```python
from build123d import *

# Parameters (mm, degrees)
F0_W     = 115
F0_H     = 47
F1_DEPTH = 183
F2_W     = 95
F2_H     = 27
F2_R     = 8
F3_DEPTH = 2
F4_W     = 20
F4_H     = 3
F5_DEPTH = 183.001
F6_W     = 3
F6_H     = 13
F7_DEPTH = 47.001


with BuildPart() as f1:
    # F0 (on Top) → F1 (new body)
    with BuildSketch(Plane.XY):
        Rectangle(F0_W, F0_H)
    extrude(amount=F1_DEPTH)

    # F2 (on face) → F3 (cut)
    with BuildSketch(Plane.XY.offset(183)):
        Rectangle(F2_W, F2_H)
        with Locations((-31, 0)):
            Circle(F2_R, mode=Mode.SUBTRACT)
        with Locations((31, 0)):
            Circle(F2_R, mode=Mode.SUBTRACT)
    extrude(amount=-F3_DEPTH, mode=Mode.SUBTRACT)

    # F4 (on face) → F5 (cut, through all)
    with BuildSketch(Plane.XY.offset(183)):
        with Locations((-37.5, 22)):
            Rectangle(F4_W, F4_H)
        with Locations((-12.5, 22)):
            Rectangle(F4_W, F4_H)
        with Locations((12.5, 22)):
            Rectangle(F4_W, F4_H)
        with Locations((37.5, 22)):
            Rectangle(F4_W, F4_H)
        with Locations((37.5, -22)):
            Rectangle(F4_W, F4_H)
        with Locations((12.5, -22)):
            Rectangle(F4_W, F4_H)
        with Locations((-12.5, -22)):
            Rectangle(F4_W, F4_H)
        with Locations((-37.5, -22)):
            Rectangle(F4_W, F4_H)
    extrude(amount=-F5_DEPTH, mode=Mode.SUBTRACT)

    # F6 (on face) → F7 (cut, through all)
    with BuildSketch(Plane.XZ.offset(23.5)):
        with Locations((-56, 171.5)):
            Rectangle(F6_W, F6_H)
        with Locations((-56, 151.5)):
            Rectangle(F6_W, F6_H)
        with Locations((-56, 131.5)):
            Rectangle(F6_W, F6_H)
        with Locations((-56, 111.5)):
            Rectangle(F6_W, F6_H)
        with Locations((-56, 91.5)):
            Rectangle(F6_W, F6_H)
        with Locations((-56, 71.5)):
            Rectangle(F6_W, F6_H)
        with Locations((-56, 51.5)):
            Rectangle(F6_W, F6_H)
        with Locations((-56, 31.5)):
            Rectangle(F6_W, F6_H)
        with Locations((-56, 11.5)):
            Rectangle(F6_W, F6_H)
        with Locations((56, 171.5)):
            Rectangle(F6_W, F6_H)
        with Locations((56, 151.5)):
            Rectangle(F6_W, F6_H)
        with Locations((56, 131.5)):
            Rectangle(F6_W, F6_H)
        with Locations((56, 111.5)):
            Rectangle(F6_W, F6_H)
        with Locations((56, 91.5)):
            Rectangle(F6_W, F6_H)
        with Locations((56, 11.5)):
            Rectangle(F6_W, F6_H)
        with Locations((56, 51.5)):
            Rectangle(F6_W, F6_H)
        with Locations((56, 71.5)):
            Rectangle(F6_W, F6_H)
        with Locations((56, 31.5)):
            Rectangle(F6_W, F6_H)
    extrude(amount=-F7_DEPTH, mode=Mode.SUBTRACT)


solid = f1.part
```
Part model, mm, in its own coordinate system. A direction names the side the tool comes from. Give positions to 0.01 mm unless a question says otherwise; leave off trailing zeros. Write each loop counter-clockwise with the first axis right and the second up, starting at its lowest first coordinate (ties: lowest second). Pieces come first, ordered by that corner, then holes. Notation, with made-up numbers: (-36.75, 71.25) -> (9.25, 71.25) arc R25 ccw to (9.25, 93.25) -> close; hole circle Ø6 at (-38.5, 8). An arc over 180 degrees is marked (long way). Put each result on its own line as item: value. Start each with the question number.
Item 1: Wall check: L1, parallel to Y at x = -5, z = 80; L2, parallel to Z at x = 14.5, y = 6.5; L3, parallel to X at y = 16.5, z = 168.5. Give the ranges that are in metal, low to high. Write a range as [from, to].
Item 2: Cut at A-A (x = -31). List the corners of the cut face in (y, z).
Item 3: Pin check, flat tips, straight feed: pin 1 Ø0.9 at (x, y) = (55.5, 8.5) entering from -Z; pin 2 Ø3 at (x, z) = (41, 159.5) entering from -Y; pin 3 Ø1.5 at (y, z) = (22, 47) entering from +X; pin 4 Ø2 at (x, z) = (-19, 182.5) entering from +Y. Stop position of each tip, or through.
Item 4: Pull direction Y, two halves, no side cores. Call faces 1 (the face through (-1, 0, 181)), 2 (the face through (-25, 23.5, 90)), 3 (the face through (54.5, 0, 131)): pulls with the +Y half, pulls with the -Y half, needs draft (parallel to the pull), parting line crosses it, or undercut.
Item 5: Which spindle directions (+Z, -Z, +X, -X, +Y, -Y) get a long thin tool onto all of the face, cutting with end or side? Do faces 4 (the face through (31, 0, 183)), 5 (the face through (-54.5, 0, 71)), 6 (the face through (54.5, 0, 91)). Say none if no direction does.
Item 6: Cut at B-B (x = 7). List the corners of the cut face in (y, z).
Answer list:
1. L1: y = [-20.5, 20.5]
1. L2: z = [0, 181]
1. L3: x = [-54.5, 54.5]
2. outline: (-20.5, 0) -> (20.5, 0) -> (20.5, 183) -> (13.5, 183) -> (13.5, 181) -> (8, 181) -> (8, 183) -> (-8, 183) -> (-8, 181) -> (-13.5, 181) -> (-13.5, 183) -> (-20.5, 183) -> close
3. pin 1: stops at z = 0
3. pin 2: stops at y = -20.5
3. pin 3: stops at x = 54.5
3. pin 4: stops at y = 20.5
4. face 1: undercut
4. face 2: pulls with the +Y half
4. face 3: needs draft
5. face 4: +Z, +X, -X, +Y, -Y
5. face 5: -X, +Y, -Y
5. face 6: +X, +Y, -Y
6. outline: (-20.5, 0) -> (20.5, 0) -> (20.5, 183) -> (13.5, 183) -> (13.5, 181) -> (-13.5, 181) -> (-13.5, 183) -> (-20.5, 183) -> close
